The model under review builds one solid part; all positions refer to its coordinate system, in mm. Face numbers are marked on the shaded views. A direction names the side the tool comes from. Round coordinates to 2 decimals unless told otherwise and drop trailing zeros. Order: outer loops, then holes, each group sorted by start corner. A loop starts at its lowest first (then second) coordinate and runs counter-clockwise, first axis right, second up. Notation, with made-up numbers: M -20.5,71.25 L -3.5,71.25 A6 ccw -3.5,77.25 Z; hole C 62.5,-6 d9. An arc over 180 degrees is marked long. Answer as a JSON object with one key per item and string values. Group by question number.
1. Add section A-A on x = 5.5. State the section outline as (y, z) points.
2. Add section C-C on y = 5.05. State the section outline as (x, z) points, and give its area (3 significant figures).
3. Machinability: for the marked faces 1, 2 and 3, which of the approach directions +Z, -Z, +X, -X, +Y, -Y give a long, thin tool a straight path to every point of the face, cutting with its end or side? Answer none if there is none.
4. Add section B-B on z = 2.5. State the section outline as (x, y) points, and give its area (3 significant figures).
5. Add section D-D on z = -0.75. State the section outline as (x, y) points, and give its area (3 significant figures).
6. To check wall thickness, follow probe 1 along X at (y, z) = (3, -4); probe 2 along X at (y, z) = (4.1, 2.5); probe 3 along Z at (x, y) = (6.3, 1.7). State the ranges of each line that lie inside material, in increasing order. Write a range as [from, to].
7. Clearance check with a flat-ended pin moving along its axis: P1, Ø1.5, axis at x = -5, y = 3, coming from the -Z side. State where the tip first meets the part, or that it passes through.
8. Mouldability with a two-part tool opening along Z and no side actions: class the marked faces 4, 5, 6 and 7 as released by +Z, released by -Z, zero draft, split by the parting line, or undercut.
```python
from build123d import *

# Parameters (mm, degrees)
SALIENTE_EXTRUIR2_DEPTH = 6
CROQUIS2_R              = 1.25
CORTAR_EXTRUIR1_DEPTH   = 10
REDONDEO1_R             = 0.1
CROQUIS3_W              = 2
CROQUIS3_H              = 3.3
CORTAR_EXTRUIR2_DEPTH   = 5
CROQUIS4_R              = 0.1
CORTAR_EXTRUIR3_DEPTH   = 6
CROQUIS5_W              = 0.5
CROQUIS5_H              = 3
CORTAR_EXTRUIR4_DEPTH   = 0.1


with BuildPart() as part:
    # Croquis1 → Saliente-Extruir2 (new body)
    with BuildSketch(Plane(origin=(0, 0, 0), x_dir=(1, 0, 0), z_dir=(0, 1, 0))):
        with BuildLine():
            Line((2.986733927, 4.5), (-10, 4.5))
            Line((-10, 4.5), (-10, -5))
            Line((-10, -5), (10, -5))
            Line((10, -5), (10, 5))
            Line((10, 5), (3.286733927, 5))
            Line((3.286733927, 5), (3.286733927, 4.8))
            ThreePointArc((3.286733927, 4.8), (3.198865961, 4.587867966), (2.986733927, 4.5))
        make_face()
    extrude(amount=SALIENTE_EXTRUIR2_DEPTH)

    # Croquis2 → Cortar-Extruir1 (cut)
    with BuildSketch(Plane(origin=(0, 6, 0), x_dir=(1, 0, 0), z_dir=(0, 1, 0))):
        with Locations(Location((-5, -2.5, 0), (0, 0, 270))):
            Circle(CROQUIS2_R)
        with Locations(Location((4.5, -2.5, 0), (0, 0, 270))):
            Circle(CROQUIS2_R)
    extrude(amount=-CORTAR_EXTRUIR1_DEPTH, mode=Mode.SUBTRACT)

    # Redondeo1
    redondeo1_edges = [part.edges().sort_by_distance(p)[0] for p in [
        (3.286733927, 3, -5),
    ]]
    fillet(redondeo1_edges, radius=REDONDEO1_R)

    # Croquis3 → Cortar-Extruir2 (cut)
    with BuildSketch(Plane(origin=(0, 0, -4.5), x_dir=(-1, 0, 0), z_dir=(0, 0, -1))):
        with Locations((-0.386733927, 3)):
            Rectangle(CROQUIS3_W, CROQUIS3_H)
    extrude(amount=-CORTAR_EXTRUIR2_DEPTH, mode=Mode.SUBTRACT)

    # Croquis4 → Cortar-Extruir3 (cut)
    with BuildSketch(Plane(origin=(0, 6, 0), x_dir=(1, 0, 0), z_dir=(0, 1, 0))):
        with Locations(Location((6.3, 4, 0), (0, 0, 270))):
            Circle(CROQUIS4_R)
    extrude(amount=-CORTAR_EXTRUIR3_DEPTH, mode=Mode.SUBTRACT)

    # Croquis5 → Cortar-Extruir4 (cut)
    with BuildSketch(Plane.XY.offset(5)):
        with Locations((-8.247200411, 3)):
            Rectangle(CROQUIS5_W, CROQUIS5_H)
        with Locations((-0.947200411, 3)):
            Rectangle(CROQUIS5_W, CROQUIS5_H)
        with Locations((8.052799589, 3)):
            Rectangle(CROQUIS5_W, CROQUIS5_H)
    extrude(amount=-CORTAR_EXTRUIR4_DEPTH, mode=Mode.SUBTRACT)


solid = part.part
```
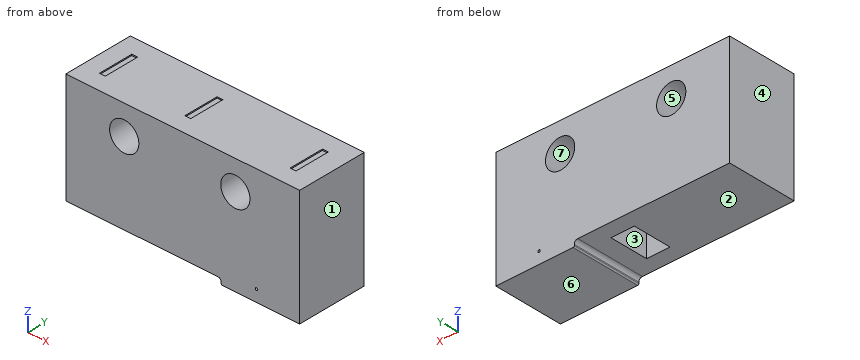
Recorded:
{
 "1": {"outline": "M 0,-5 L 6,-5 L 6,1.75 L 0,1.75 Z; M 0,3.25 L 6,3.25 L 6,5 L 0,5 Z"},
 "2": {"outline": "M -10,-4.5 L 2.99,-4.5 A0.3 cw 3.29,-4.8 L 3.29,-4.9 A0.1 ccw 3.39,-5 L 10,-5 L 10,5 L -10,5 Z; hole C -5,2.5 d2.5; hole C 4.5,2.5 d2.5; hole C 6.3,-4 d0.2", "area": "184 mm²"},
 "3": {"face 1": "+Z, -Z, +X, +Y, -Y", "face 2": "-Z, -X, +Y, -Y", "face 3": "-Z"},
 "4": {"outline": "M -10,0 L -6.25,0 L -6.25,6 L -10,6 Z; M -3.75,0 L 3.25,0 L 3.25,6 L -3.75,6 Z; M 5.75,0 L 10,0 L 10,6 L 5.75,6 Z", "area": "90.0 mm²"},
 "5": {"outline": "M -10,0 L 10,0 L 10,6 L -10,6 Z; hole M -0.61,1.35 L 1.39,1.35 L 1.39,4.65 L -0.61,4.65 Z", "area": "113 mm²"},
 "6": {"probe 1": "x = [-10, -0.61], [1.39, 6.2], [6.4, 10]", "probe 2": "x = [-10, -6.25], [-3.75, 3.25], [5.75, 10]", "probe 3": "z = [-5, -4.1], [-3.9, 5]"},
 "7": {"P1": "stops at z = -4.5"},
 "8": {"face 4": "zero draft", "face 5": "undercut", "face 6": "released by -Z", "face 7": "undercut"}
}
